Check sheet for the modelled part. Datum: model origin and axes. Units: mm. Face numbers are marked on the shaded views. Give positions to 0.01 mm unless a question says otherwise; leave off trailing zeros. Order: outer loops, then holes, each group sorted by start corner. A loop starts at its lowest first (then second) coordinate and runs counter-clockwise, first axis right, second up. Notation, with made-up numbers: (21.5, 77) -> (71.5, 77) arc R21 ccw to (71.5, 101) -> close; hole circle Ø7 at (7.25, 47). An arc over 180 degrees is marked (long way). One line per question, with ' | ' between items.
```python
from build123d import *

# Parameters (mm, degrees)
BOSS_EXTRUDE1_DEPTH     = 30
SKETCH4_R               = 2.5
CUT_EXTRUDE1_DEPTH      = 1
CUT_EXTRUDE1_DEPTH_BACK = 46
SKETCH6_W               = 75
SKETCH6_H               = 25
CUT_EXTRUDE3_DEPTH      = 31
SKETCH7_R               = 6
SKETCH7_R_2             = 2.5
BOSS_EXTRUDE2_DEPTH     = 2.5
SKETCH8_R               = 6
SKETCH8_R_2             = 2.5
BOSS_EXTRUDE3_DEPTH     = 5


with BuildPart() as part:
    # Sketch1 → Boss-Extrude1 (new body)
    with BuildSketch(Plane(origin=(0, 0, 0), x_dir=(1, 0, 0), z_dir=(0, 1, 0))):
        with BuildLine():
            Line((-30, 15), (30, 15))
            ThreePointArc((30, 15), (45, 0), (30, -15))
            Line((30, -15), (-30, -15))
            ThreePointArc((-30, -15), (-45, 0), (-30, 15))
        make_face()
    extrude(amount=BOSS_EXTRUDE1_DEPTH)

    # Sketch4 → Cut-Extrude1 (cut, two sides)
    with BuildSketch(Plane(origin=(0, 30, 0), x_dir=(1, 0, 0), z_dir=(0, 1, 0))) as cut_extrude1_sk:
        with Locations((-30, 0)):
            Circle(SKETCH4_R)
    extrude(amount=CUT_EXTRUDE1_DEPTH, mode=Mode.SUBTRACT)
    extrude(cut_extrude1_sk.sketch, amount=-CUT_EXTRUDE1_DEPTH_BACK, mode=Mode.SUBTRACT)

    # Sketch6 → Cut-Extrude3 (cut, through all)
    with BuildSketch(Plane.XY.offset(15)):
        with Locations((-7.5, 15)):
            Rectangle(SKETCH6_W, SKETCH6_H)
    extrude(amount=-CUT_EXTRUDE3_DEPTH, mode=Mode.SUBTRACT)

    # Sketch7 → Boss-Extrude2 (add)
    with BuildSketch(Plane(origin=(0, 30, 0), x_dir=(1, 0, 0), z_dir=(0, 1, 0))):
        with Locations((-30, 0)):
            Circle(SKETCH7_R)
        with Locations((-30, 0)):
            Circle(SKETCH7_R_2, mode=Mode.SUBTRACT)
    extrude(amount=BOSS_EXTRUDE2_DEPTH)

    # Sketch8 → Boss-Extrude3 (add)
    with BuildSketch(Plane.XZ):
        with Locations((-30, 0)):
            Circle(SKETCH8_R)
        with Locations((-30, 0)):
            Circle(SKETCH8_R_2, mode=Mode.SUBTRACT)
    extrude(amount=-BOSS_EXTRUDE3_DEPTH)


solid = part.part
```
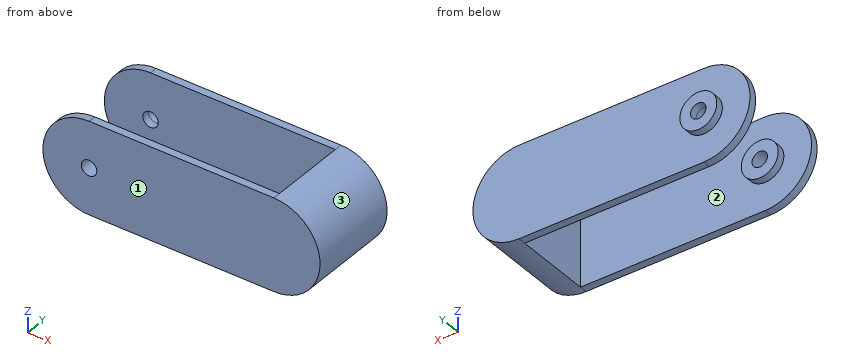
Q1. Section check D-D (y = 3.5). Enter the section's corners in (x, z), and give its area (3 significant figures).
Result sheet:
outline: circle Ø12 at (-30, 0); (30, -15) arc R15 ccw to (30, 15) -> close; hole circle Ø5 at (-30, 0) | area: 447 mm2
Q2. Section check A-A (x = 14.5). Enter the section's corners in (y, z), and give its area (3 significant figures).
Result sheet:
outline: (0, -15) -> (2.5, -15) -> (2.5, 15) -> (0, 15) -> close; (27.5, -15) -> (30, -15) -> (30, 15) -> (27.5, 15) -> close | area: 150 mm2
Q3. Mould release check, pull along Y, two halves, no side actions. Record for the marked faces 1, 2 and 3: pulls with the +Y half, pulls with the -Y half, needs draft (parallel to the pull), parting line crosses it, or undercut.
Result sheet:
face 1: pulls with the -Y half | face 2: undercut | face 3: needs draft
Q4. Section check C-C (y = 29). Enter the section's corners in (x, z).
Result sheet:
outline: (-30, -15) -> (30, -15) arc R15 ccw to (30, 15) -> (-30, 15) arc R15 ccw to start; hole circle Ø5 at (-30, 0)
Q5. Section check B-B (z = 0). Enter the section's corners in (x, y), and give its area (3 significant figures).
Result sheet:
outline: (-45, 0) -> (-32.5, 0) -> (-32.5, 5) -> (-36, 5) -> (-36, 2.5) -> (-45, 2.5) -> close; (-45, 27.5) -> (-32.5, 27.5) -> (-32.5, 32.5) -> (-36, 32.5) -> (-36, 30) -> (-45, 30) -> close; (-27.5, 0) -> (45, 0) -> (45, 30) -> (-24, 30) -> (-24, 32.5) -> (-27.5, 32.5) -> (-27.5, 27.5) -> (30, 27.5) -> (30, 2.5) -> (-24, 2.5) -> (-24, 5) -> (-27.5, 5) -> close | area: 835 mm2
Q6. Depth check by flat-ended pin: pin 1 Ø10 at (y, z) = (20.5, 9.5) entering from +X; pin 2 Ø7.5 at (y, z) = (16.5, -5) entering from -X; pin 3 Ø3 at (x, z) = (-30, 0) entering from -Y; pin 4 Ø2 at (y, z) = (17.5, 8) entering from +X. Enter the tip coordinate at first touch or a pass-through.
Result sheet:
pin 1: stops at x = 44.31 | pin 2: stops at x = 30 | pin 3: passes through | pin 4: stops at x = 43.27
Q7. Thickness scan on line 1 (X direction, y = 28.1, z = 0); line 2 (Y direction, x = -14, z = 1.5); line 3 (Z direction, x = -30, y = 31.95). Record the ranges inside material, lowest first.
Result sheet:
line 1: x = -45 to -32.5, -27.5 to 45 | line 2: y = 0 to 2.5, 27.5 to 30 | line 3: z = -6 to -2.5, 2.5 to 6
